Job drawing, mm, ordinate dimensions from the low corner. One solid piece. A direction names the side the tool comes from. Round coordinates to 2 decimals unless told otherwise and drop trailing zeros. Order: outer loops, then holes, each group sorted by start corner. A loop starts at its lowest first (then second) coordinate and runs counter-clockwise, first axis right, second up. Notation, with made-up numbers: (47, 57.25) -> (58, 57.25) arc R14 ccw to (58, 71.25) -> close; hole circle Ø1 at (42, 3.25). An arc over 180 degrees is marked (long way). Write item = value, one per line.
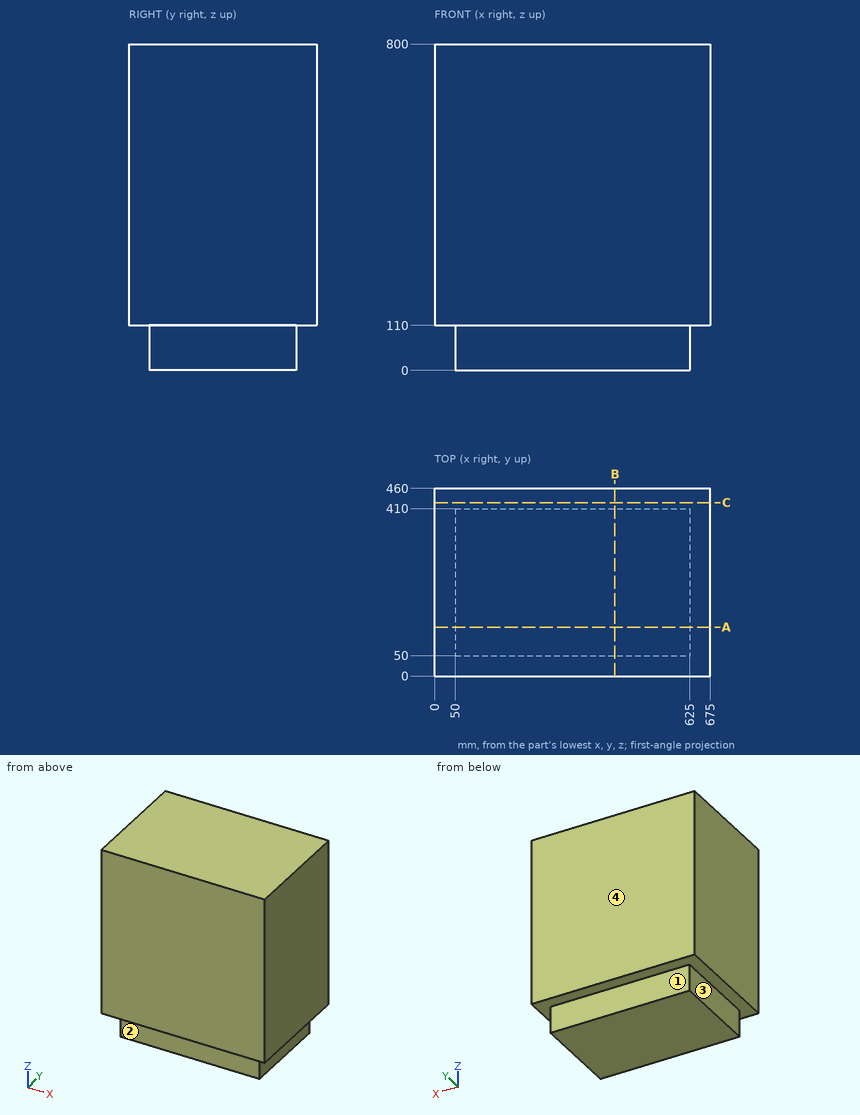
Q1. Which spindle directions (+Z, -Z, +X, -X, +Y, -Y) get a long thin tool onto all of the face, cutting with end or side? Do the marked faces 1, 2, 3 and 4. Say none if no direction does.
Check values:
face_1 = -Z, +X, -X, +Y
face_2 = -Z, +X, -X, -Y
face_3 = -Z, -X, +Y, -Y
face_4 = +Z, -Z, +X, -X, +Y
Q2. Cut at B-B, the plane x = 442. List the corners of the cut face in (y, z).
Check values:
outline = (0, 110) -> (50, 110) -> (50, 0) -> (410, 0) -> (410, 110) -> (460, 110) -> (460, 800) -> (0, 800) -> close
Q3. Probe probe 1 along Z at (x, y) = (197.5, 46.5); probe 2 along X at (y, z) = (369.5, 86); probe 3 along Y at (x, z) = (364, 87). List the from-to ranges inside material, lowest first.
Check values:
probe_1 = 110 to 800
probe_2 = 50 to 625
probe_3 = 50 to 410
Q4. Cut at C-C, the plane y = 425. List the corners of the cut face in (x, z).
Check values:
outline = (0, 110) -> (675, 110) -> (675, 800) -> (0, 800) -> close
Q5. Cut at A-A, the plane y = 120. List the corners of the cut face in (x, z), and give its area (3 significant figures).
Check values:
outline = (0, 110) -> (50, 110) -> (50, 0) -> (625, 0) -> (625, 110) -> (675, 110) -> (675, 800) -> (0, 800) -> close
area = 529,000 mm²
Q6. Flat gauge pins, fed straight in: pin 1 (6 mm diameter, centred on x = 123, z = 91.5, fed in from +Y); pin 2 (1 mm diameter, centred on x = 425.5, y = 181.5, fed in from -Z). Where does each tip first touch, or does it go through?
Check values:
pin_1 = 410
pin_2 = 0
